```python
from build123d import *

# Parameters (mm, degrees)
F0_W           = 106.68
F0_H           = 10.16
F2_DEPTH       = 50.8
F2_DEPTH_BACK  = 50.8
F1_W           = 50.8
F1_H           = 40.64
F4_DEPTH       = 10.16
F5_D           = 10.3124
F5_CSINK_D     = 19.8374
F5_CSINK_ANGLE = 82
F6_R           = 15.24


with BuildPart() as f2:
    # F0 (on Front) → F2 (new body, two sides)
    with BuildSketch(Plane.XZ) as f2_sk:
        Polygon((0, 76.2), (0, 10.16), (10.16, 10.16), (10.16, 86.36), (0, 86.36), align=None)
        Polygon((10.16, 10.16), (0, 10.16), (0, 0), (101.6, 0), (101.6, 10.16), align=None)
        with Locations((-53.34, 81.28)):
            Rectangle(F0_W, F0_H)
    extrude(amount=-F2_DEPTH)
    extrude(f2_sk.sketch, amount=F2_DEPTH_BACK)

    # F1 (on Top) → F4 (cut, through all)
    with BuildSketch(Plane.XY):
        with Locations((76.2, 0)):
            Rectangle(F1_W, F1_H)
    extrude(amount=F4_DEPTH, mode=Mode.SUBTRACT)

    # F5 (through all)
    with Locations(Plane.XY.offset(86.36)):
        with Locations((-71.12, -20.32), (-71.12, 20.32)):
            CounterSinkHole(F5_D / 2, F5_CSINK_D / 2, counter_sink_angle=F5_CSINK_ANGLE)

    # F6
    f6_edges = [f2.edges().sort_by_distance(p)[0] for p in [
        (50.8, 20.32, 5.08),
        (50.8, -20.32, 5.08),
    ]]
    fillet(f6_edges, radius=F6_R)


solid = f2.part
```
Can you work these out from the model? Positions are in its coordinate system, mm. A direction names the side the tool comes from. Coordinates: 2 decimals unless noted, no trailing zeros. Loops run counter-clockwise (first coordinate to the right, second up) from the corner with the lowest first, then second, coordinate; pieces in that order, holes last.
Item 1: Suppose I cut it at D-D (z = 59.5). Please give me the cut outline in (x, y).
Answers below:
outline: (0, -50.8) - (10.16, -50.8) - (10.16, 50.8) - (0, 50.8) - close
Item 2: If we mould it in two halves opening along X, with no side actions, what happens to faces 1 (the face through (-65.97, -20.09, 78.51)), 2 (the face through (55.38, 15.97, 5.15)), 3 (the face through (5, 50.8, 47))? For each: released by +X, released by -X, zero draft, split by the parting line, or undercut.
Answers below:
face 1: undercut
face 2: released by +X
face 3: zero draft
Item 3: I'm going to push flat-ended pins straight in: pin 1 (11 mm diameter, centred on y = 1, z = 7, fed in from +X); pin 2 (6 mm diameter, centred on x = 71.5, y = 34.5, fed in from +Z); pin 3 (1.5 mm diameter, centred on y = 36.5, z = 35, fed in from -X). Where does each tip first touch, or does it pass through?
Answers below:
pin 1: stops at x = 50.87
pin 2: stops at z = 10.16
pin 3: stops at x = 0
Item 4: Suppose I cut it at A-A (x = -71.12). Please give me the cut outline in (y, z).
Answers below:
outline: (-50.8, 76.2) - (-25.48, 76.2) - (-25.48, 80.88) - (-30.24, 86.36) - (-50.8, 86.36) - close; (-15.16, 76.2) - (15.16, 76.2) - (15.16, 80.88) - (10.4, 86.36) - (-10.4, 86.36) - (-15.16, 80.88) - close; (25.48, 76.2) - (50.8, 76.2) - (50.8, 86.36) - (30.24, 86.36) - (25.48, 80.88) - close
Item 5: Suppose I cut it at B-B (y = -35.5). Please give me the cut outline in (x, z), then the cut area to 3 significant figures.
Answers below:
outline: (-106.68, 76.2) - (0, 76.2) - (0, 0) - (101.6, 0) - (101.6, 10.16) - (10.16, 10.16) - (10.16, 86.36) - (-106.68, 86.36) - close
area: 2,890 mm2
Item 6: Suppose I cut it at C-C (x = 61.5). Please give me the cut outline in (y, z), then the cut area to 3 significant figures.
Answers below:
outline: (-50.8, 0) - (-19.63, 0) - (-19.63, 10.16) - (-50.8, 10.16) - close; (19.63, 0) - (50.8, 0) - (50.8, 10.16) - (19.63, 10.16) - close
area: 633 mm2
Item 7: Please list where these lines run through material, in increasing order: L1, parallel to Y at x = -71.12, z = 79.9; L2, parallel to X at y = -20.32, z = 79.55; L3, parallel to X at y = 4, z = 66.
Answers below:
L1: y = -50.8 to -25.48, -15.16 to 15.16, 25.48 to 50.8
L2: x = -106.68 to -76.28, -65.96 to 10.16
L3: x = 0 to 10.16
Item 8: Which directions (+Z, -Z, +X, -X, +Y, -Y) give clear straight access to the entire face, cutting with the end or side of a thin tool? Please do faces 4 (the face through (-106.68, 1, 81)), 5 (the face through (84, -20.32, 5)), 6 (the face through (10.16, 1, 48)).
Answers below:
face 4: +Z, -Z, -X, +Y, -Y
face 5: +Z, -Z, +X
face 6: +Z, +X, +Y, -Y
